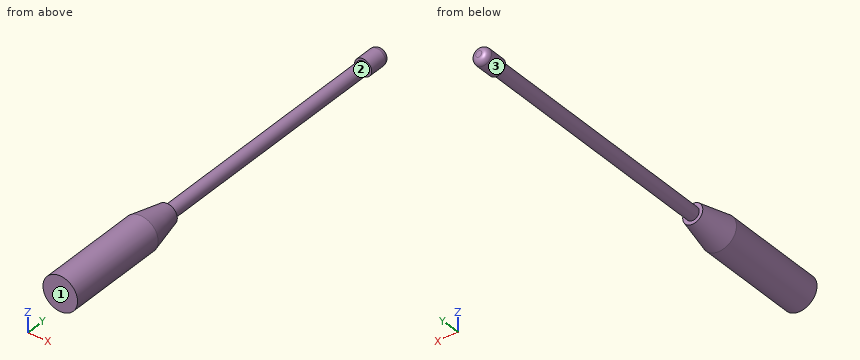
```python
from build123d import *

# Parameters (mm, degrees)
SKETCH1_R           = 2.38125
BOSS_EXTRUDE1_DEPTH = 152.4
SKETCH2_R           = 6.35
BOSS_EXTRUDE2_DEPTH = 50.8
CHAMFER1_SIZE       = 12.54
CHAMFER1_SIZE2      = 2.665459283
SKETCH3_R           = 3.14325
BOSS_EXTRUDE3_DEPTH = 8.636
FILLET1_R           = 2.032


with BuildPart() as part:
    # Sketch1 → Boss-Extrude1 (new body)
    with BuildSketch(Plane(origin=(0, 0, 0), x_dir=(1, 0, 0), z_dir=(0, 1, 0))):
        Circle(SKETCH1_R)
    extrude(amount=BOSS_EXTRUDE1_DEPTH)

    # Sketch2 → Boss-Extrude2 (add)
    with BuildSketch(Plane(origin=(0, 0, 0), x_dir=(1, 0, 0), z_dir=(0, 1, 0))):
        Circle(SKETCH2_R)
    extrude(amount=BOSS_EXTRUDE2_DEPTH)

    # Chamfer1
    chamfer1_edges = [part.edges().sort_by_distance(p)[0] for p in [
        (-6.35, 50.8, 0),
    ]]
    chamfer1_side = [part.faces().sort_by_distance(p)[0] for p in [
        (-6.35, 25.4, 0),
    ]]
    chamfer(chamfer1_edges, length=CHAMFER1_SIZE, length2=CHAMFER1_SIZE2, reference=chamfer1_side[0])

    # Sketch3 → Boss-Extrude3 (add)
    with BuildSketch(Plane(origin=(0, 152.4, 0), x_dir=(1, 0, 0), z_dir=(0, 1, 0))):
        Circle(SKETCH3_R)
    extrude(amount=-BOSS_EXTRUDE3_DEPTH)

    # Fillet1
    fillet1_edges = [part.edges().sort_by_distance(p)[0] for p in [
        (-3.14325, 152.4, 0),
    ]]
    fillet(fillet1_edges, radius=FILLET1_R)


solid = part.part
```
Verification items for the finished model (mm, model axes). Face numbers are marked on the shaded views. A direction names the side the tool comes from. Round coordinates to 2 decimals unless told otherwise and drop trailing zeros. Write each loop counter-clockwise with the first axis right and the second up, starting at its lowest first coordinate (ties: lowest second). Pieces come first, ordered by that corner, then holes. Notation, with made-up numbers: (20, 3.5) - (58, 3.5) arc R18 ccw to (58, 32.5) - close; hole circle Ø4 at (37.25, -3.75). An arc over 180 degrees is marked (long way). Answer as a JSON object with one key per item and string values. Group by question number.
Q1. Section check A-A, the plane y = 136. Enter the section's corners in (x, z), plus the area to 3 significant figures.
Q2. Thickness scan on line 1 (Y direction, x = -1.25, z = -3.25); line 2 (Z direction, x = 5.5, y = 31); line 3 (Z direction, x = 0, y = 103.5). Record the ranges inside material, lowest first.
Q3. Tool access check on the marked faces 1, 2 and 3. Record the directions out of +Z, -Z, +X, -X, +Y, -Y that give a thin tool (end or side, any length) a straight path to the whole face; none if there is none.
Q4. Go/stop test with flat-tipped pins: pin 1 Ø4 at (x, y) = (-1.5, 133) entering from +Z; pin 2 Ø5 at (y, z) = (94, 2) entering from +X; pin 3 Ø4 at (y, z) = (68.5, 3.5) entering from +X. Record where each tip stops, or that it passes through.
Found:
{
 "1": {"outline": "circle Ø4.76 at (0, 0)", "area": "17.8 mm^2"},
 "2": {"line 1": "y = 0 to 50.8", "line 2": "z = -3.17 to 3.17", "line 3": "z = -2.38 to 2.38"},
 "3": {"face 1": "+Z, -Z, +X, -X, -Y", "face 2": "none", "face 3": "+Y"},
 "4": {"pin 1": "stops at z = 2.38", "pin 2": "stops at x = 2.38", "pin 3": "stops at x = 1.85"}
}
